from build123d import *

# Parameters (mm, degrees)
SKETCH1_W           = 15
SKETCH1_H           = 100
BOSS_EXTRUDE1_DEPTH = 15


with BuildPart() as part:
    # Sketch1 → Boss-Extrude1 (new body)
    with BuildSketch(Plane.XY):
        Polygon((0, 0), (0, 600), (250, 850), (500, 600), (500, 0), align=None)
        with Locations((37.5, 460)):
            Rectangle(SKETCH1_W, SKETCH1_H, mode=Mode.SUBTRACT)
        with Locations((462.5, 460)):
            Rectangle(SKETCH1_W, SKETCH1_H, mode=Mode.SUBTRACT)
        with Locations((462.5, 140)):
            Rectangle(SKETCH1_W, SKETCH1_H, mode=Mode.SUBTRACT)
        with Locations((37.5, 140)):
            Rectangle(SKETCH1_W, SKETCH1_H, mode=Mode.SUBTRACT)
        Polygon((61.819805153, 640.606601718), (72.426406871, 630), (125.45941546, 683.033008589), (114.852813742, 693.639610307), align=None, mode=Mode.SUBTRACT)
        Polygon((166.966991411, 724.54058454), (156.360389693, 735.147186258), (209.393398282, 788.180194847), (220, 777.573593129), align=None, mode=Mode.SUBTRACT)
        Polygon((280, 777.573593129), (333.033008589, 724.54058454), (343.639610307, 735.147186258), (290.606601718, 788.180194847), align=None, mode=Mode.SUBTRACT)
        Polygon((374.54058454, 683.033008589), (385.147186258, 693.639610307), (438.180194847, 640.606601718), (427.573593129, 630), align=None, mode=Mode.SUBTRACT)
    extrude(amount=BOSS_EXTRUDE1_DEPTH)


solid = part.part
Source: CAD feature listing. Evaluate the final solid. Frame: model axes, mm. A direction names the side the tool comes from. Give positions to 0.01 mm unless a question says otherwise; leave off trailing zeros. Write each loop counter-clockwise with the first axis right and the second up, starting at its lowest first coordinate (ties: lowest second). Pieces come first, ordered by that corner, then holes. Notation, with made-up numbers: M 40,64.25 L 86,64.25 A21 ccw 86,86.25 Z; hole C 36,-0.5 d5. An arc over 180 degrees is marked long. Return JSON: item names as keys, results as strings. Group by question number.
1) Set-up query: faces 5 (the face through (470, 459, 7)), 6 (the face through (0, 296, 7)). Return all of +Z, -Z, +X, -X, +Y, -Y with unobstructed straight access to the full face (end or side cutting, diameter ignored); none if empty.
2) Cut plane A-A, the plane y = 490. Output: boundary loops of the cut face in (x, z).
3) Pin query (flat end, axial travel): P1, Ø3, axis at y = 764, z = 2.5, coming from the -X side; P2, Ø4.5, axis at x = 459, z = 10, coming from the -Y side; P3, Ø4.5, axis at x = 35.5, z = 7.5, coming from the +Y side; P4, Ø4.5, axis at x = 460.5, z = 9, coming from the +Y side. Return the tip coordinate at first contact, or that it passes through.
4) Cut plane B-B, the plane x = 301.5. Output: boundary loops of the cut face in (y, z).
5) Cut plane C-C, the plane z = 7.5. Give the number of separate pieces and of enclosed holes in the cut face, plus the area to 3 significant figures.
6) Material intervals for line 1 along X through (y, z) = (456, 13); line 2 along Y through (x, z) = (38, 6); line 3 along X through (y, z) = (693, 8.25), sorted ascending. Write a range as [from, to].
7) Pull-direction query (X, two-part tool) for faces 1 (the face through (123, 723, 7)), 2 (the face through (254, 337, 15)), 3 (the face through (37, 190, 7)), 4 (the face through (30, 139, 7)); classes: pulls with the +X half, pulls with the -X half, needs draft (parallel to the pull), parting line crosses it, or undercut.
Recorded:
{
 "1": {"face 5": "+Z, -Z", "face 6": "+Z, -Z, -X, +Y, -Y"},
 "2": {"outline": "M 0,0 L 30,0 L 30,15 L 0,15 Z; M 45,0 L 455,0 L 455,15 L 45,15 Z; M 470,0 L 500,0 L 500,15 L 470,15 Z"},
 "3": {"P1": "stops at x = 162.5", "P2": "stops at y = 0", "P3": "stops at y = 637.75", "P4": "stops at y = 641.75"},
 "4": {"outline": "M 0,0 L 756.07,0 L 756.07,15 L 0,15 Z; M 777.29,0 L 798.5,0 L 798.5,15 L 777.29,15 Z"},
 "5": {"separate pieces": "1", "enclosed holes": "8", "area": "352,000 mm²"},
 "6": {"line 1": "x = [0, 30], [45, 455], [470, 500]", "line 2": "y = [0, 90], [190, 410], [510, 638]", "line 3": "x = [93, 114.21], [115.49, 384.51], [385.79, 407]"},
 "7": {"face 1": "pulls with the -X half", "face 2": "needs draft", "face 3": "undercut", "face 4": "undercut"}
}
